from build123d import *

# Parameters (mm, degrees)
BOSS_EXTRUDE2_DEPTH = 1524
CHAMFER1_SIZE       = 2.54


with BuildPart() as part:
    # Sketch3 → Boss-Extrude2 (new body)
    with BuildSketch(Plane(origin=(0, 0, 0), x_dir=(0, 0, -1), z_dir=(1, 0, 0))):
        Polygon((0, 0), (0, 254), (304.8, 254), (304.8, 508), (609.6, 508), (609.6, 762), (914.4, 762), (914.4, 1016), (1219.2, 1016), (1219.2, 1270), (1524, 1270), (1524, 1524), (1828.8, 1524), (1828.8, 1270), (1828.8, 1016), (1524, 1016), (1524, 762), (1219.2, 762), (1219.2, 508), (914.4, 508), (914.4, 254), (609.6, 254), (609.6, 0), align=None)
    extrude(amount=BOSS_EXTRUDE2_DEPTH)

    # Chamfer1
    chamfer1_edges = [part.edges().sort_by_distance(p)[0] for p in [
        (1524, 254, -762),
        (1524, 381, -914.4),
        (1524, 508, -1066.8),
        (1524, 635, -1219.2),
        (0, 127, 0),
        (0, 254, -152.4),
        (0, 381, -304.8),
        (0, 508, -457.2),
        (0, 635, -609.6),
        (0, 762, -762),
        (1524, 762, -1371.6),
        (0, 889, -914.4),
        (0, 1016, -1066.8),
        (0, 1143, -1219.2),
        (0, 1270, -1371.6),
        (0, 1397, -1524),
        (0, 1524, -1676.4),
        (0, 1270, -1828.8),
        (1524, 889, -1524),
        (0, 1016, -1676.4),
        (0, 889, -1524),
        (0, 762, -1371.6),
        (0, 635, -1219.2),
        (0, 508, -1066.8),
        (0, 381, -914.4),
        (0, 254, -762),
        (1524, 1016, -1676.4),
        (0, 127, -609.6),
        (0, 0, -304.8),
        (1524, 1270, -1828.8),
        (762, 0, 0),
        (762, 254, 0),
        (762, 254, -304.8),
        (762, 508, -304.8),
        (762, 508, -609.6),
        (762, 762, -609.6),
        (762, 762, -914.4),
        (762, 1016, -914.4),
        (762, 1016, -1219.2),
        (762, 1270, -1219.2),
        (762, 1270, -1524),
        (1524, 1524, -1676.4),
        (762, 1524, -1524),
        (762, 1524, -1828.8),
        (762, 1016, -1828.8),
        (762, 1016, -1524),
        (762, 762, -1524),
        (762, 762, -1219.2),
        (762, 508, -1219.2),
        (762, 508, -914.4),
        (762, 254, -914.4),
        (762, 254, -609.6),
        (762, 0, -609.6),
        (1524, 0, -304.8),
        (1524, 1397, -1524),
        (1524, 1270, -1371.6),
        (1524, 1143, -1219.2),
        (1524, 1016, -1066.8),
        (1524, 889, -914.4),
        (1524, 762, -762),
        (1524, 635, -609.6),
        (1524, 508, -457.2),
        (1524, 381, -304.8),
        (1524, 254, -152.4),
        (1524, 127, -609.6),
        (1524, 127, 0),
    ]]
    chamfer(chamfer1_edges, length=CHAMFER1_SIZE)


solid = part.part
Geometry check sheet. Reference: the model listing, model coordinates, mm. A direction names the side the tool comes from. Round coordinates to 2 decimals unless told otherwise and drop trailing zeros. Write each loop counter-clockwise with the first axis right and the second up, starting at its lowest first coordinate (ties: lowest second). Pieces come first, ordered by that corner, then holes. Notation, with made-up numbers: (-1, -24.75) - (39, -24.75) arc R26 ccw to (39, -0.75) - close; hole circle Ø3 at (-28.5, 51.5). An arc over 180 degrees is marked (long way). One line per item, written item: value.
1. Cross-section at A-A on y = 335.5. Record the boundary of the cut face in (x, z).
The answers:
outline: (0, -911.86) - (2.54, -914.4) - (1521.46, -914.4) - (1524, -911.86) - (1524, -307.34) - (1521.46, -304.8) - (2.54, -304.8) - (0, -307.34) - close
2. Cross-section at B-B on z = -1679. Record the boundary of the cut face in (x, y), and give its area (3 significant figures).
The answers:
outline: (0, 1018.54) - (2.54, 1016) - (1521.46, 1016) - (1524, 1018.54) - (1524, 1521.46) - (1521.46, 1524) - (2.54, 1524) - (0, 1521.46) - close
area: 774,000 mm^2
3. Depth check by flat-ended pin: pin 1 Ø3 at (x, y) = (1156, 826.5) entering from +Z; pin 2 Ø4 at (x, y) = (851, 1328) entering from +Z; pin 3 Ø2 at (x, z) = (968, -1452) entering from -Y; pin 4 Ø10 at (y, z) = (809, -1079.5) entering from -X. Enter the tip coordinate at first touch or a pass-through.
The answers:
pin 1: stops at z = -914.4
pin 2: stops at z = -1524
pin 3: stops at y = 762
pin 4: stops at x = 0
4. Set-up check for faces 1 (the face through (751, 762, -760)), 2 (the face through (751, 637, -1219.2)), 3 (the face through (751, 1524, -1674)): record each of +Z, -Z, +X, -X, +Y, -Y from which the full face is reachable in a straight line by a thin tool's end or side.
The answers:
face 1: +Z, +X, -X, +Y
face 2: -Z, +X, -X, -Y
face 3: +Z, -Z, +X, -X, +Y
5. Scan lines: L1, parallel to Y at x = 965.5, z = -168.5; L2, parallel to Z at x = 1320.5, y = 240.5; L3, parallel to Z at x = 473, y = 927.5. Record each from-to range of solid material in increasing order.
The answers:
L1: y = 0 to 254
L2: z = -609.6 to 0
L3: z = -1524 to -914.4
